Verification items for the finished model (mm, model axes). A direction names the side the tool comes from. Round coordinates to 2 decimals unless told otherwise and drop trailing zeros. Loops run counter-clockwise (first coordinate to the right, second up) from the corner with the lowest first, then second, coordinate; pieces in that order, holes last.
from build123d import *

# Parameters (mm, degrees)
SKETCH_1_W          = 30
SKETCH_1_H          = 15
SKETCH_1_R          = 1.5
EXTRUDE_1_DEPTH     = 11
SKETCH_2_R          = 1.5
CUT_EXTRUDE_1_DEPTH = 20
SKETCH_3_W          = 12
SKETCH_3_H          = 5
CUT_EXTRUDE_2_DEPTH = 20
SKETCH_5_W          = 18
SKETCH_5_H          = 8
CUT_EXTRUDE_3_DEPTH = 10
CHAMFER_1_SIZE      = 5


with BuildPart() as part:
    # 草图1 → 凸台-拉伸1 (new body)
    with BuildSketch(Plane.XY):
        with Locations((15, 7.5)):
            Rectangle(SKETCH_1_W, SKETCH_1_H)
        with Locations((8, 5)):
            Circle(SKETCH_1_R, mode=Mode.SUBTRACT)
    extrude(amount=EXTRUDE_1_DEPTH)

    # 草图2 → 切除-拉伸1 (cut)
    with BuildSketch(Plane.XZ):
        with Locations(Location((25, 4, 0), (0, 0, 270))):
            Circle(SKETCH_2_R)
        with Locations(Location((17, 4, 0), (0, 0, 270))):
            Circle(SKETCH_2_R)
    extrude(amount=-CUT_EXTRUDE_1_DEPTH, mode=Mode.SUBTRACT)

    # 草图3 → 切除-拉伸2 (cut)
    with BuildSketch(Plane.XZ):
        with Locations((6, 2.5)):
            Rectangle(SKETCH_3_W, SKETCH_3_H)
    extrude(amount=-CUT_EXTRUDE_2_DEPTH, mode=Mode.SUBTRACT)

    # 草图5 → 切除-拉伸3 (cut)
    with BuildSketch(Plane.XZ):
        with Locations((21, 4)):
            Rectangle(SKETCH_5_W, SKETCH_5_H)
    extrude(amount=-CUT_EXTRUDE_3_DEPTH, mode=Mode.SUBTRACT)

    # 倒角1
    chamfer_1_edges = [part.edges().sort_by_distance(p)[0] for p in [
        (12, 12.5, 5),
    ]]
    chamfer(chamfer_1_edges, length=CHAMFER_1_SIZE - 0.0001)  # a hair under: the kernel refuses the full size


solid = part.part
1. Release check for a two-part mould opening along X. For faces 1 (the face through (21, 13, 0)), 2 (the face through (10, 12, 2)), 3 (the face through (18.265, 12.465, 3.194)) record: released by +X, released by -X, zero draft, split by the parting line, or undercut.
2. Section check A-A (x = 25). Enter the section's corners in (y, z).
3. Tool access check on faces 4 (the face through (5, 7, 5)), 5 (the face through (12, 5, 6)), 6 (the face through (0, 7, 8)). Record the directions out of +Z, -Z, +X, -X, +Y, -Y that give a thin tool (end or side, any length) a straight path to the whole face; none if there is none.
4. Section check D-D (y = 7.75). Enter the section's corners in (x, z).
5. Section check B-B (y = 5). Enter the section's corners in (x, z), then the cut area to 3 significant figures.
6. Section check C-C (z = 4). Enter the section's corners in (x, y).
7. Scan lines: L1, parallel to X at y = 12.3, z = 4; L2, parallel to X at y = 5, z = 8.7; L3, parallel to Z at x = 11.5, y = 1.5. Record each from-to range of solid material in increasing order.
8. Gauge pin test, flat ends, axial feed: P1, Ø5, axis at x = 17, z = 4, coming from the -Y side; P2, Ø5, axis at x = 22, y = 2, coming from the -Z side; P3, Ø1.5, axis at y = 7, z = 6.5, coming from the +X side. Record the tip position at first contact, or that the pin passes through.
Taken from the geometry:
1. face 1: zero draft
1. face 2: released by -X
1. face 3: undercut
2. outline: (0, 8) - (10, 8) - (10, 5.5) - (15, 5.5) - (15, 11) - (0, 11) - close; (10, 0) - (15, 0) - (15, 2.5) - (10, 2.5) - close
3. face 4: -Z, -X, -Y
3. face 5: -Z, +X, -Y
3. face 6: +Z, -Z, -X, +Y, -Y
4. outline: (0, 5) - (12, 5) - (12, 8) - (30, 8) - (30, 11) - (0, 11) - close
5. outline: (0, 5) - (6.5, 5) - (6.5, 11) - (0, 11) - close; (9.5, 5) - (12, 5) - (12, 8) - (30, 8) - (30, 11) - (9.5, 11) - close
5. area: 108 mm2
6. outline: (8, 10) - (15.5, 10) - (15.5, 15) - (8, 15) - close; (18.5, 10) - (23.5, 10) - (23.5, 15) - (18.5, 15) - close; (26.5, 10) - (30, 10) - (30, 15) - (26.5, 15) - close
7. L1: x = 8 to 15.5, 18.5 to 23.5, 26.5 to 30
7. L2: x = 0 to 6.5, 9.5 to 30
7. L3: z = 5 to 11
8. P1: stops at y = 10
8. P2: stops at z = 8
8. P3: stops at x = 12
